```python
from build123d import *

# Parameters (mm, degrees)
SKETCH1_R           = 17.318879346
SKETCH1_R_2         = 5.411731441
BOSS_EXTRUDE1_DEPTH = 6
BOSS_EXTRUDE2_DEPTH = 7.5
SKETCH2_W           = 11
SKETCH2_H           = 12.996419178
CUT_EXTRUDE1_DEPTH  = 26
FILLET1_R           = 1


with BuildPart() as part:
    # Sketch1 → Boss-Extrude1 (new body, symmetric)
    with BuildSketch(Plane.XY):
        Circle(SKETCH1_R)
        Circle(SKETCH1_R_2, mode=Mode.SUBTRACT)
    extrude(amount=BOSS_EXTRUDE1_DEPTH, both=True)

    # Sketch1_3 → Boss-Extrude2 (add, symmetric)
    with BuildSketch(Plane.XY):
        with BuildLine():
            Line((-43.539982068, -8.498209589), (-15.090527346, -8.498209589))
            ThreePointArc((-15.090527346, -8.498209589), (-17.318879346, 0), (-15.090527346, 8.498209589))
            Line((-15.090527346, 8.498209589), (-43.539982068, 8.498209589))
            Line((-43.539982068, 8.498209589), (-43.539982068, -8.498209589))
        make_face()
    extrude(amount=BOSS_EXTRUDE2_DEPTH, both=True)

    # Sketch2 → Cut-Extrude1 (cut)
    with BuildSketch(Plane.ZY.offset(43.539982068)):
        Rectangle(SKETCH2_W, SKETCH2_H)
    extrude(amount=-CUT_EXTRUDE1_DEPTH, mode=Mode.SUBTRACT)

    # Fillet1
    fillet1_edges = [part.edges().sort_by_distance(p)[0] for p in [
        (-29.315254707, 8.498209589, -7.5),
        (-29.315254707, -8.498209589, 7.5),
        (-29.315254707, 8.498209589, 7.5),
        (-29.315254707, -8.498209589, -7.5),
    ]]
    fillet(fillet1_edges, radius=FILLET1_R)


solid = part.part
```
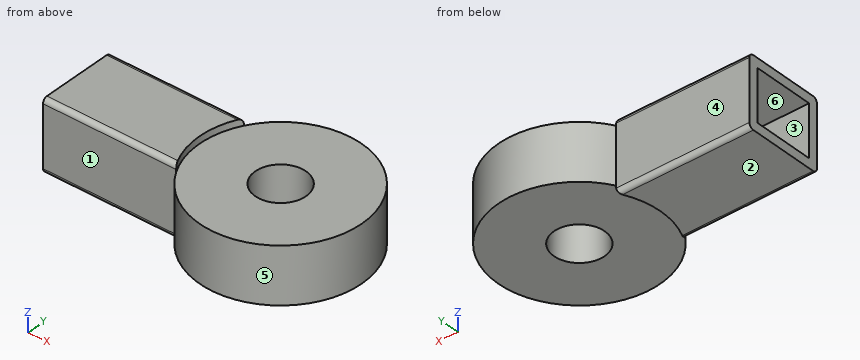
Geometry check sheet. Reference: the model listing, model coordinates, mm. Face numbers are marked on the shaded views. A direction names the side the tool comes from. Coordinates: 2 decimals unless noted, no trailing zeros. Order: outer loops, then holes, each group sorted by start corner. A loop starts at its lowest first (then second) coordinate and runs counter-clockwise, first axis right, second up.
Item 1: Mould release check, pull along Y, two halves, no side actions. Record for the marked faces 4, 5 and 6: released by +Y, released by -Y, zero draft, split by the parting line, or undercut.
Item 2: Section check A-A (x = 0). Enter the section's corners in (y, z).
Item 3: Depth check by flat-ended pin: pin 1 (1.5 mm diameter, centred on x = 9.5, y = -10.5, fed in from -Z); pin 2 (3.5 mm diameter, centred on y = -2.5, z = -1, fed in from -X); pin 3 (12 mm diameter, centred on x = 3, y = 6.5, fed in from +Z); pin 4 (9.5 mm diameter, centred on x = 0, y = 0, fed in from +Z). Enter the tip coordinate at first touch or a pass-through.
Item 4: Section check C-C (x = -36.5). Enter the section's corners in (y, z).
Item 5: Tool access check on the marked faces 1, 2 and 3. Record the directions out of +Z, -Z, +X, -X, +Y, -Y that give a thin tool (end or side, any length) a straight path to the whole face; none if there is none.
Item 6: Scan lines: line 1 along Y through (x, z) = (-31, 5); line 2 along Y through (x, z) = (0, 3.25); line 3 along Z through (x, y) = (12, 1). Record each from-to range of solid material in increasing order.
Item 7: Section check B-B (z = 3.25). Enter the section's corners in (x, y), plus the area to 3 significant figures.
Item 8: Section check D-D (y = 2.5). Enter the section's corners in (x, z), plus the area to 3 significant figures.
Check sheet entries:
1. face 4: released by +Y
1. face 5: split by the parting line
1. face 6: undercut
2. outline: (-17.32, -6) - (-5.41, -6) - (-5.41, 6) - (-17.32, 6) - close; (5.41, -6) - (17.32, -6) - (17.32, 6) - (5.41, 6) - close
3. pin 1: stops at z = -6
3. pin 2: stops at x = -17.54
3. pin 3: stops at z = 6
3. pin 4: passes through
4. outline: (-8.5, -6.5) arc R1 ccw to (-7.5, -7.5) - (7.5, -7.5) arc R1 ccw to (8.5, -6.5) - (8.5, 6.5) arc R1 ccw to (7.5, 7.5) - (-7.5, 7.5) arc R1 ccw to (-8.5, 6.5) - close; hole (-6.5, -5.5) - (6.5, -5.5) - (6.5, 5.5) - (-6.5, 5.5) - close
5. face 1: +Z, -Z, -X, -Y
5. face 2: -Z, +X, -X, +Y, -Y
5. face 3: -X
6. line 1: y = -8.5 to -6.5, 6.5 to 8.5
6. line 2: y = -17.32 to -5.41, 5.41 to 17.32
6. line 3: z = -6 to 6
7. outline: (-43.54, -8.5) - (-15.09, -8.5) arc R17.32 ccw (long way) to (-15.09, 8.5) - (-43.54, 8.5) - (-43.54, 6.5) - (-17.54, 6.5) - (-17.54, -6.5) - (-43.54, -6.5) - close; hole circle Ø10.82 at (0, 0)
7. area: 970 mm2
8. outline: (-43.54, -7.5) - (-17.14, -7.5) - (-17.14, -6) - (-4.8, -6) - (-4.8, 6) - (-17.14, 6) - (-17.14, 7.5) - (-43.54, 7.5) - (-43.54, 5.5) - (-17.54, 5.5) - (-17.54, -5.5) - (-43.54, -5.5) - close; (4.8, -6) - (17.14, -6) - (17.14, 6) - (4.8, 6) - close
8. area: 406 mm2
